```python
from build123d import *

# Parameters (mm, degrees)
SALIENTE_EXTRUIR1_DEPTH = 9
CROQUIS2_R              = 1.875
CORTAR_EXTRUIR1_DEPTH   = 8.5
CROQUIS2_3_R            = 3.5
CROQUIS2_3_R_2          = 1.875
CORTAR_EXTRUIR2_DEPTH   = 2.8


with BuildPart() as part:
    # Croquis1 → Saliente-Extruir1 (new body)
    with BuildSketch(Plane(origin=(0, 0, 0), x_dir=(1, 0, 0), z_dir=(0, 1, 0))):
        with BuildLine():
            Line((17.88854382, 16), (20, 16))
            ThreePointArc((20, 16), (23.818961075, 9.415789574), (25.53429067, 2))
            Line((25.53429067, 2), (43.53429067, 2))
            Line((43.53429067, 2), (43.53429067, 9.5))
            Line((43.53429067, 9.5), (32.645826686, 9.5))
            ThreePointArc((32.645826686, 9.5), (0, 34), (-32.645826686, 9.5))
            Line((-32.645826686, 9.5), (-43.53429067, 9.5))
            Line((-43.53429067, 9.5), (-43.53429067, 2))
            Line((-43.53429067, 2), (-25.53429067, 2))
            ThreePointArc((-25.53429067, 2), (-23.818961075, 9.415789574), (-20, 16))
            Line((-20, 16), (-17.88854382, 16))
            ThreePointArc((-17.88854382, 16), (0, 24), (17.88854382, 16))
        make_face()
    extrude(amount=SALIENTE_EXTRUIR1_DEPTH)

    # Croquis2 → Cortar-Extruir1 (cut, through all)
    with BuildSketch(Plane(origin=(0, 0, -9.5), x_dir=(-1, 0, 0), z_dir=(0, 0, -1))):
        with Locations((37.645, 4.5)):
            Circle(CROQUIS2_R)
        with Locations((-37.645, 4.5)):
            Circle(CROQUIS2_R)
    extrude(amount=-CORTAR_EXTRUIR1_DEPTH, mode=Mode.SUBTRACT)

    # Croquis2_3 → Cortar-Extruir2 (cut)
    with BuildSketch(Plane(origin=(0, 0, -9.5), x_dir=(-1, 0, 0), z_dir=(0, 0, -1))):
        with Locations((-37.645, 4.5)):
            Circle(CROQUIS2_3_R)
        with Locations((-37.645, 4.5)):
            Circle(CROQUIS2_3_R_2, mode=Mode.SUBTRACT)
        with Locations((37.645, 4.5)):
            Circle(CROQUIS2_3_R)
        with Locations((37.645, 4.5)):
            Circle(CROQUIS2_3_R_2, mode=Mode.SUBTRACT)
    extrude(amount=-CORTAR_EXTRUIR2_DEPTH, mode=Mode.SUBTRACT)


solid = part.part
```
Input: part model. Units: mm. Frame: model coordinates. A direction names the side the tool comes from. Coordinates: 2 decimals unless noted, no trailing zeros. Write each loop counter-clockwise with the first axis right and the second up, starting at its lowest first coordinate (ties: lowest second). Pieces come first, ordered by that corner, then holes.
1) Section C-C on z = -21. Output: boundary loops of the cut face in (x, y), and give its area (3 significant figures).
2) Section A-A on y = 4.5. Output: boundary loops of the cut face in (x, z) (1 decimal), and give its area (3 significant figures).
3) Material intervals for line 1 along Z through (x, y) = (-37, 7.5); line 2 along X through (y, z) = (3.5, -11.5); line 3 along Z through (x, y) = (0, 8.5), sorted ascending.
4) Set-up query: faces 4 (the flat face through (-39.2, 3, -6.7)), 5 (the flat face through (-19, 4, -16)), 6 (the flat face through (-42, 4, -9.5)). Return all of +Z, -Z, +X, -X, +Y, -Y with unobstructed straight access to the full face (end or side cutting, diameter ignored); none if empty.
5) Pin query (flat end, axial travel): pin 1 Ø2.5 at (x, y) = (19.5, 6) entering from +Z; pin 2 Ø10 at (x, z) = (-32.5, -29.5) entering from -Y; pin 3 Ø1.7 at (x, y) = (-19.5, 6) entering from +Z; pin 4 Ø3 at (x, y) = (9.5, 6) entering from -Z. Return the tip coordinate at first contact, or that it passes through.
6) Mould query, pull axis X, two halves, no side actions, for faces 1 (the flat face through (19, 4, -16)), 2 (the flat face through (43.534, 4, -6)), 3 (the flat face through (-3, 9, -24)). Classes: pulls with the +X half, pulls with the -X half, needs draft (parallel to the pull), parting line crosses it, or undercut.
7) Section B-B on z = -5. Output: boundary loops of the cut face in (x, y) (3 decimals).
8) Section D-D on x = -6. Output: boundary loops of the cut face in (y, z), and give its area (3 significant figures).
Check result:
1. outline: (-26.74, 0) - (-11.62, 0) - (-11.62, 9) - (-26.74, 9) - close; (11.62, 0) - (26.74, 0) - (26.74, 9) - (11.62, 9) - close
1. area: 272 mm2
2. outline: (-43.5, -9.5) - (-41.1, -9.5) - (-41.1, -6.7) - (-39.5, -6.7) - (-39.5, -2) - (-43.5, -2) - close; (-35.8, -6.7) - (-34.1, -6.7) - (-34.1, -9.5) - (-32.6, -9.5) arc R34 ccw to (32.6, -9.5) - (34.1, -9.5) - (34.1, -6.7) - (35.8, -6.7) - (35.8, -2) - (25.5, -2) arc R25.6 cw to (20, -16) - (17.9, -16) arc R24 cw to (-17.9, -16) - (-20, -16) arc R25.6 cw to (-25.5, -2) - (-35.8, -2) - close; (39.5, -6.7) - (41.1, -6.7) - (41.1, -9.5) - (43.5, -9.5) - (43.5, -2) - (39.5, -2) - close
2. area: 898 mm2
3. line 1: z = -6.7 to -2
3. line 2: x = -32 to -22.89, 22.89 to 32
3. line 3: z = -34 to -24
4. face 4: -Z
4. face 5: +Z, +Y, -Y
4. face 6: -Z, -X, +Y, -Y
5. pin 1: stops at z = -15.01
5. pin 2: passes through
5. pin 3: stops at z = -15.55
5. pin 4: stops at z = -33.05
6. face 1: undercut
6. face 2: pulls with the +X half
6. face 3: needs draft
7. outline: (-43.534, 0) - (-25.12, 0) - (-25.12, 9) - (-43.534, 9) - close; (25.12, 0) - (43.534, 0) - (43.534, 9) - (25.12, 9) - close; hole circle Ø3.75 at (-37.645, 4.5); hole circle Ø3.75 at (37.645, 4.5)
8. outline: (0, -33.47) - (9, -33.47) - (9, -23.24) - (0, -23.24) - close
8. area: 92.1 mm2
